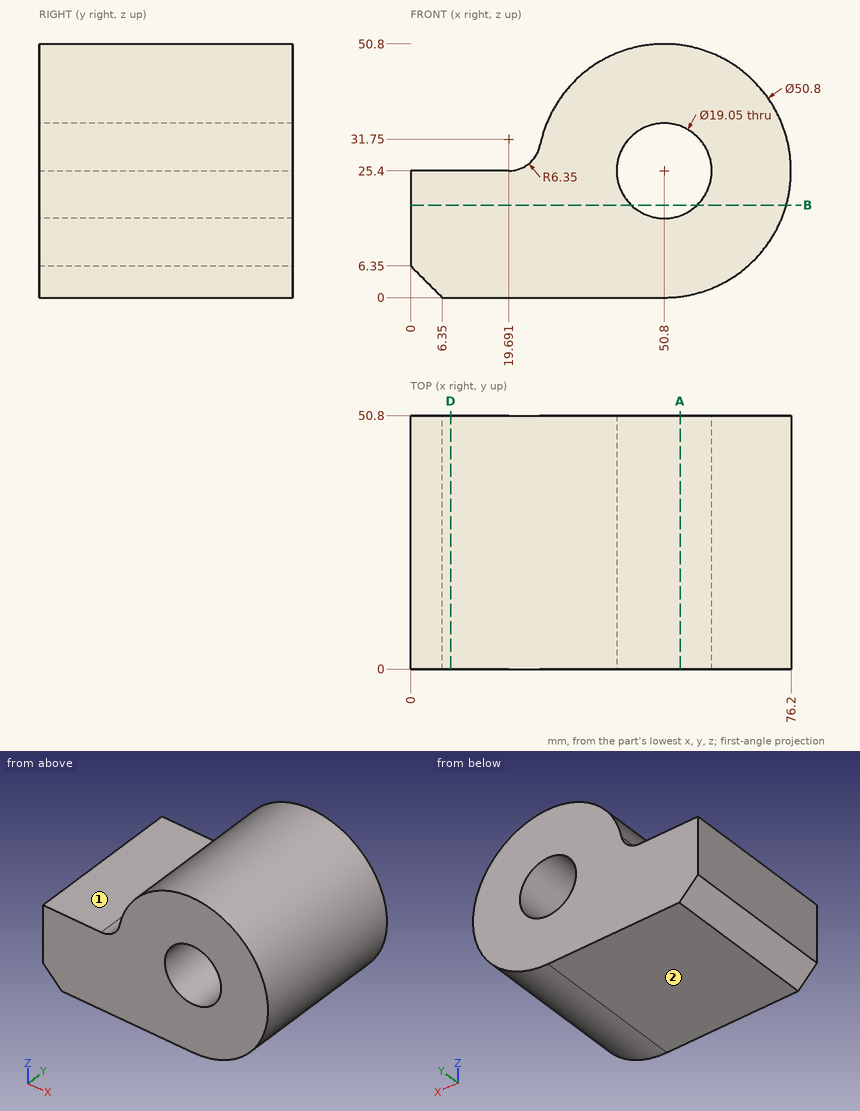
Here's the drawing with two shaded views (mm, measured from the low corner). I have some questions. A direction names the side the tool comes from. Coordinates: 2 decimals unless noted, no trailing zeros. Loops run counter-clockwise (first coordinate to the right, second up) from the corner with the lowest first, then second, coordinate; pieces in that order, holes last. Notation, with made-up numbers: (37.25, 45.5) -> (68.25, 45.5) arc R23 ccw to (68.25, 57.5) -> close; hole circle Ø4 at (25, -23). An arc over 180 degrees is marked (long way). Answer as a JSON object with one key per item and string values.
1) For the marked faces 1 and 2, which set-ups out of +Z, -Z, +X, -X, +Y, -Y let a thin tool reach every point of the face, with its end or its side?
Results:
{"face 1": "+Z, -X, +Y, -Y", "face 2": "-Z, +X, -X, +Y, -Y"}
2) Imagine slicing it at D-D (x = 8). Please give me the cut outline in (y, z), then the cut area to 3 significant figures.
Results:
{"outline": "(0, 0) -> (50.8, 0) -> (50.8, 25.4) -> (0, 25.4) -> close", "area": "1,290 mm^2"}
3) Imagine slicing it at A-A (x = 54). Please give me the cut outline in (y, z).
Results:
{"outline": "(0, 0.2) -> (50.8, 0.2) -> (50.8, 16.43) -> (0, 16.43) -> close; (0, 34.37) -> (50.8, 34.37) -> (50.8, 50.6) -> (0, 50.6) -> close"}
4) If I drill on line 1 (Z direction, x = 50.8, y = 18.5) (1 decimal); line 2 (X direction, y = 25, z = 25); line 3 (Z direction, x = 7, y = 11), over which ranges is the centre line in solid material (lowest first)?
Results:
{"line 1": "z = 0 to 15.9, 34.9 to 50.8", "line 2": "x = 0 to 41.28, 60.32 to 76.2", "line 3": "z = 0 to 25.4"}
5) Imagine slicing it at B-B (z = 18.5). Please give me the cut outline in (x, y) (1 decimal).
Results:
{"outline": "(0, 0) -> (44.2, 0) -> (44.2, 50.8) -> (0, 50.8) -> close; (57.4, 0) -> (75.2, 0) -> (75.2, 50.8) -> (57.4, 50.8) -> close"}
6) For P1, Ø8, axis at y = 21, z = 10.5, coming from the +X side; P2, Ø12, axis at x = 15, y = 10, coming from the +Z side; P3, Ø12, axis at y = 34, z = 34, coming from the +X side, each with a flat end and sliding along its axis, tell me the tip position at first contact or that it passes through.
Results:
{"P1": "stops at x = 73.74", "P2": "stops at z = 25.54", "P3": "stops at x = 76.07"}
